Job drawing, mm, ordinate dimensions from the low corner. One solid piece. A direction names the side the tool comes from. Give positions to 0.01 mm unless a question says otherwise; leave off trailing zeros. Write each loop counter-clockwise with the first axis right and the second up, starting at its lowest first coordinate (ties: lowest second). Pieces come first, ordered by that corner, then holes. Notation, with made-up numbers: M 53.25,78 L 106.25,78 A16 cw 106.25,90 Z; hole C 8.25,41 d4. An arc over 180 degrees is marked long. Answer as CSV lines item,"result". Start each with the question number.
1) Tool access for the marked faces 1, 2, 3 and 4: list every direction of +Z, -Z, +X, -X, +Y, -Y with a clear straight run to the whole face (end or side of a thin tool).
2) Pin check, flat tips, straight feed: pin 1 Ø1.6 at (x, z) = (4.5, 34) entering from -Y; pin 2 Ø0.6 at (y, z) = (1, 20.5) entering from -X; pin 3 Ø1.5 at (x, y) = (11, 18.5) entering from -Z. Stop position of each tip, or through.
3) Slice it at A-A, the plane z = 9. Give the cut face in (x, y).
4) Slice it at B-B, the plane y = 31. Give the cut face in (x, z), plus the area to 3 significant figures.
5) Wall check: line 1 along Z through (x, y) = (15.5, 7.5); line 2 along X through (y, z) = (3.5, 49). Give the ranges that are in metal, low to high. Write a range as from..to.
6) Slice it at C-C, the plane x = 18.5. Give the cut face in (y, z).
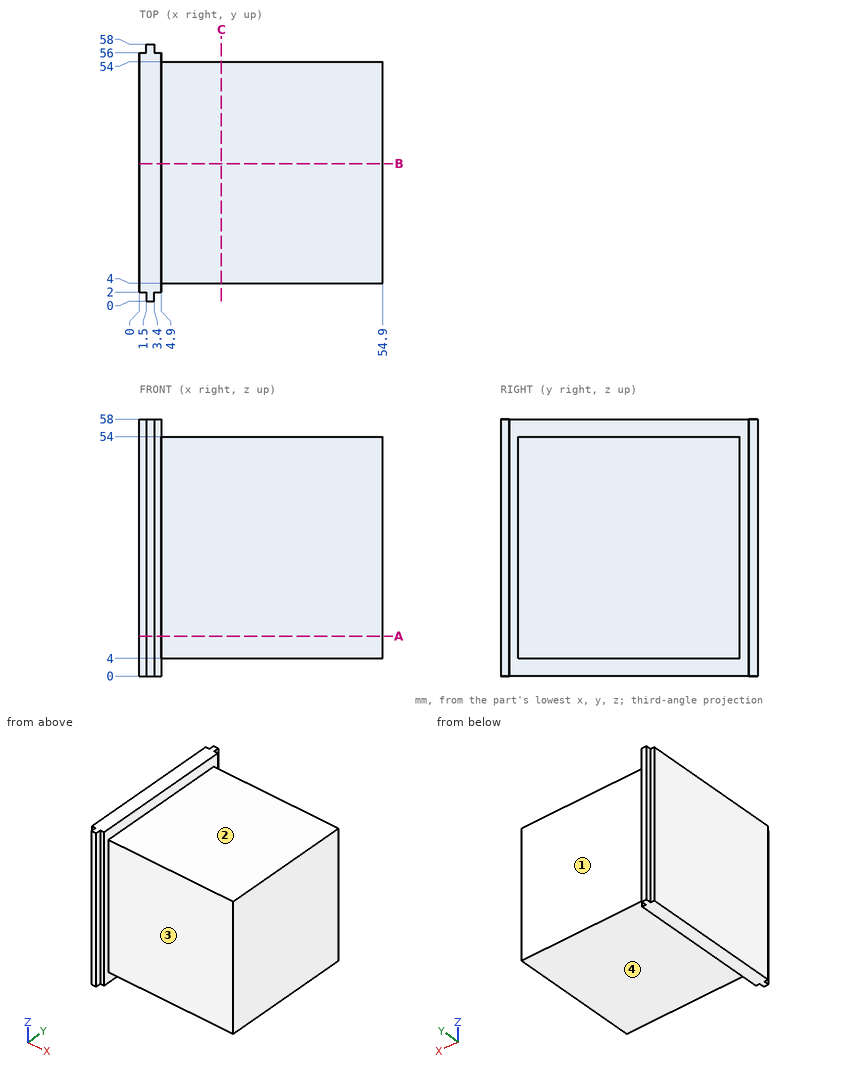
Found:
1,face 1,"+Z, -Z, +X, +Y"
1,face 2,"+Z, +X, +Y, -Y"
1,face 3,"+Z, -Z, +X, -Y"
1,face 4,"-Z, +X, +Y, -Y"
2,pin 1,"y = 2"
2,pin 2,"x = 1.5"
2,pin 3,"z = 4"
3,outline,"M 0,2 L 1.5,2 L 1.5,0 L 3.4,0 L 3.4,2 L 4.9,2 L 4.9,4 L 54.9,4 L 54.9,54 L 4.9,54 L 4.9,56 L 3.4,56 L 3.4,58 L 1.5,58 L 1.5,56 L 0,56 Z"
4,outline,"M 0,0 L 4.9,0 L 4.9,4 L 54.9,4 L 54.9,54 L 4.9,54 L 4.9,58 L 0,58 Z"
4,area,"2,780 mm²"
5,line 1,"4..54"
5,line 2,"0..4.9"
6,outline,"M 4,4 L 54,4 L 54,54 L 4,54 Z"
